Autodesk Inventor part; units mm, degrees
ref_plane "YZ Plane" through (0, 0, 0) normal (1, 0, 0) x (0, 1, 0)
ref_plane "XZ Plane" through (0, 0, 0) normal (0, 1, 0) x (-1, 0, 0)
ref_plane "XY Plane" through (0, 0, 0) normal (0, 0, 1) x (1, 0, 0)
sketch "Szkic1" plane through (0, 0, 0) normal (0, 0, 1) x (1, 0, 0)
  line L0 (-63, 0) -> (63, 0)
  line L1 (0, -28.7) -> (0, 28.7)
  line L2 (-45, -20.5) -> (45, -20.5)
  line L3 (45, -20.5) -> (45, 20.5)
  line L4 (45, 20.5) -> (-45, 20.5)
  line L5 (-45, 20.5) -> (-45, -20.5)
  line L6 (-45, -20.5) -> (45, 20.5) construction
  line L7 (45, -20.5) -> (-45, 20.5) construction
  point P0 (0, 0)
  dimension "d0" = 90
  dimension "d1" = 41
extrude "Wyciągnięcie proste1" add sketch "Szkic1" along normal blind 1.5
sketch "Szkic2" plane through (45, -20.5, 0) normal (1, 0, 0) x (0, 0, -1)
  line L0 (0, 0) -> (0, 41)
  line L1 (0, 41) -> (-1.5, 41)
  line L2 (-1.5, 0) -> (-1.5, 41)
  line L3 (0, 0) -> (-1.5, 0)
  line L4 (0, 0) -> (-1.5, 0)
  line L5 (0, 0) -> (-1.5, 1.5)
  line L6 (-1.5, 0) -> (-1.5, 41)
  line L7 (0, 41) -> (-1.5, 41)
  line L8 (0, 41) -> (-1.5, 40.454)
  point P0 (0, 20.5)
  dimension "d4" = 45
  dimension "d5" = 70
extrude "Wyciągnięcie proste2" cut sketch "Szkic2" against normal blind 90 contours L3 L2 L5 | L8 L2 L1
sketch "Szkic3" plane through (0, 0, 0) normal (0, 0, -1) x (-1, 0, 0)
  line L0 (45, 20.5) -> (45, -20.5)
  line L1 (-45, 20.5) -> (45, 20.5)
  point P0 (0, 0)
  point P1 (40.5, 0.5)
  dimension "d8" = 4.5
  dimension "d9" = 20
hole "Otwór1" at (-40.5, 0.5, 0) direction (0, 0, 1) diameter 3 depth 4
sketch "Szkic4" plane through (0, 0, 1.5) normal (0, 0, 1) x (1, 0, 0)
  circle A0 centre (-40.5, 0.5) radius 1.5
  line L0 (-45, -19) -> (45, -19)
  line L1 (45, -19) -> (45, 19.954)
  line L2 (45, 19.954) -> (-45, 19.954)
  line L3 (-45, 19.954) -> (-45, -19)
  line L4 (0, -28.7) -> (0, 28.7)
  line L5 (-63, 0) -> (63, 0)
  line L6 (-45, -20.5) -> (45, -20.5)
  line L7 (-45, -20.5) -> (-45, -19)
  line L8 (45, -19) -> (45, -20.5)
  line L9 (-3, -20.5) -> (-17, -20.5)
  line L10 (-17, -20.5) -> (-17, -10.5)
  line L11 (-17, -10.5) -> (-3, -10.5)
  line L12 (-3, -10.5) -> (-3, -20.5)
  line L13 (-22, -20.5) -> (-42, -20.5)
  line L14 (-42, -20.5) -> (-42, -10.5)
  line L15 (-42, -10.5) -> (-22, -10.5)
  line L16 (-22, -10.5) -> (-22, -20.5)
  point P0 (0, 0)
  point P1 (-42, -20.5)
  dimension "d17" = 14
  dimension "d18" = 20
  dimension "d19" = 10
  dimension "d20" = 10
  dimension "d21" = 5
  dimension "d22" = 3
extrude "Wyciągnięcie proste3" cut sketch "Szkic4" against normal blind 5 contours L14 L15 L16 L0 | L0 L16 L6 L14 | L12 L6 L10 L0 | L0 L10 L11 L12
mirror "Odbij2" about plane through (0, 0, 0) normal (1, 0, 0) of "Wyciągnięcie proste3", "Otwór1"
properties part number "pług_część2" material "Stal"
Geometry check sheet. Reference: the model listing, model coordinates, mm. A direction names the side the tool comes from. Give positions to 0.01 mm unless a question says otherwise; leave off trailing zeros. Order: outer loops, then holes, each group sorted by start corner. A loop starts at its lowest first (then second) coordinate and runs counter-clockwise, first axis right, second up.
1. Section check A-A, the plane y = 0.5. Enter the section's corners in (x, z), and give its area (3 significant figures).
2. Gauge pin test, flat ends, axial feed: pin 1 Ø1.5 at (x, y) = (-9, -13) entering from +Z; pin 2 Ø1.5 at (x, y) = (-5.5, 4.5) entering from -Z. Record the tip position at first contact, or that the pin passes through.
3. Release check for a two-part mould opening along X. For faces 1 (the face through (-45, 0, 1)), 2 (the face through (-1, 5, 1.5)), 3 (the face through (-22, -15, 1)), 4 (the face through (45, 0, 1)) record: pulls with the +X half, pulls with the -X half, needs draft (parallel to the pull), parting line crosses it, or undercut.
4. Section check B-B, the plane x = 40.5. Enter the section's corners in (y, z).
5. Section check D-D, the plane x = -31.5. Enter the section's corners in (y, z), and give its area (3 significant figures).
6. Thickness scan on L1, parallel to X at y = -17, z = 0.2; L2, parallel to X at y = 0.5, z = 0.8; L3, parallel to X at y = 1.5, z = 0.6. Record the ranges inside material, lowest first.
7. Access from +Z, -Z, +X, -X, +Y, -Y to the whole of each face (thin tool, end or side, straight path). Record for faces 5 (the face through (0, -19.8, 0.7)), 6 (the face through (3, -16, 1)).
8. Section check C-C, the plane z = 0.75. Enter the section's corners in (x, y), and give its area (3 significant figures).
Values follow:
1. outline: (-45, 0) - (-42, 0) - (-42, 1.5) - (-45, 1.5) - close; (-39, 0) - (39, 0) - (39, 1.5) - (-39, 1.5) - close; (42, 0) - (45, 0) - (45, 1.5) - (42, 1.5) - close
1. area: 126 mm2
2. pin 1: passes through
2. pin 2: stops at z = 0
3. face 1: pulls with the -X half
3. face 2: needs draft
3. face 3: undercut
3. face 4: pulls with the +X half
4. outline: (-10.5, 0) - (-1, 0) - (-1, 1.5) - (-10.5, 1.5) - close; (2, 0) - (20.5, 0) - (19.95, 1.5) - (2, 1.5) - close
5. outline: (-10.5, 0) - (20.5, 0) - (19.95, 1.5) - (-10.5, 1.5) - close
5. area: 46.1 mm2
6. L1: x = -45 to -42, -22 to -17, -3 to 3, 17 to 22, 42 to 45
6. L2: x = -45 to -42, -39 to 39, 42 to 45
6. L3: x = -45 to -41.62, -39.38 to 39.38, 41.62 to 45
7. face 5: +Z, +X, -X, -Y
7. face 6: +Z, -Z, -Y
8. outline: (-45, -19.75) - (-42, -19.75) - (-42, -10.5) - (-22, -10.5) - (-22, -19.75) - (-17, -19.75) - (-17, -10.5) - (-3, -10.5) - (-3, -19.75) - (3, -19.75) - (3, -10.5) - (17, -10.5) - (17, -19.75) - (22, -19.75) - (22, -10.5) - (42, -10.5) - (42, -19.75) - (45, -19.75) - (45, 20.23) - (-45, 20.23) - close; hole circle Ø3 at (-40.5, 0.5); hole circle Ø3 at (40.5, 0.5)
8. area: 2,950 mm2
